```python
from build123d import *

# Parameters (mm, degrees)
SKETCH_1_W          = 250
SKETCH_1_H          = 250
SKETCH_1_W_2        = 206
SKETCH_1_H_2        = 84
EXTRUDE_1_DEPTH     = 5.8
CUT_EXTRUDE_1_REACH = 355.601
SKETCH_2_W          = 47.2
SKETCH_2_H          = 5.8
SKETCH_2_W_2        = 5.8
SKETCH_2_H_2        = 53


with BuildPart() as part:
    # Эскиз1 → Бобышка-Вытянуть1 (new body)
    with BuildSketch(Plane(origin=(0, 0, 0), x_dir=(1, 0, 0), z_dir=(0, 1, 0))):
        with Locations((125, 125)):
            Rectangle(SKETCH_1_W, SKETCH_1_H)
        with Locations((125, 186)):
            Rectangle(SKETCH_1_W_2, SKETCH_1_H_2, mode=Mode.SUBTRACT)
        with Locations((125, 64)):
            Rectangle(SKETCH_1_W_2, SKETCH_1_H_2, mode=Mode.SUBTRACT)
    extrude(amount=EXTRUDE_1_DEPTH)

    # Эскиз2 → Вырез-Вытянуть1 (cut, up to next)
    with BuildSketch(Plane(origin=(0, 5.8, 0), x_dir=(1, 0, 0), z_dir=(0, 1, 0)), mode=Mode.PRIVATE) as cut_extrude_1_sk1:
        with Locations((77.4, 2.9)):
            Rectangle(SKETCH_2_W, SKETCH_2_H)
    cut_extrude_1_tool1 = extrude(cut_extrude_1_sk1.sketch, amount=-CUT_EXTRUDE_1_REACH, mode=Mode.PRIVATE) & part.part
    # Эскиз2 → Вырез-Вытянуть1 (cut, up to next)
    with BuildSketch(Plane(origin=(0, 5.8, 0), x_dir=(1, 0, 0), z_dir=(0, 1, 0)), mode=Mode.PRIVATE) as cut_extrude_1_sk2:
        with Locations((77.4, 125)):
            Rectangle(SKETCH_2_W, SKETCH_2_H)
    cut_extrude_1_tool2 = extrude(cut_extrude_1_sk2.sketch, amount=-CUT_EXTRUDE_1_REACH, mode=Mode.PRIVATE) & part.part
    # Эскиз2 → Вырез-Вытянуть1 (cut, up to next)
    with BuildSketch(Plane(origin=(0, 5.8, 0), x_dir=(1, 0, 0), z_dir=(0, 1, 0)), mode=Mode.PRIVATE) as cut_extrude_1_sk3:
        with Locations((77.4, 247.1)):
            Rectangle(SKETCH_2_W, SKETCH_2_H)
    cut_extrude_1_tool3 = extrude(cut_extrude_1_sk3.sketch, amount=-CUT_EXTRUDE_1_REACH, mode=Mode.PRIVATE) & part.part
    # Эскиз2 → Вырез-Вытянуть1 (cut, up to next)
    with BuildSketch(Plane(origin=(0, 5.8, 0), x_dir=(1, 0, 0), z_dir=(0, 1, 0)), mode=Mode.PRIVATE) as cut_extrude_1_sk4:
        with Locations((2.9, 175.5)):
            Rectangle(SKETCH_2_W_2, SKETCH_2_H_2)
    cut_extrude_1_tool4 = extrude(cut_extrude_1_sk4.sketch, amount=-CUT_EXTRUDE_1_REACH, mode=Mode.PRIVATE) & part.part
    # Эскиз2 → Вырез-Вытянуть1 (cut, up to next)
    with BuildSketch(Plane(origin=(0, 5.8, 0), x_dir=(1, 0, 0), z_dir=(0, 1, 0)), mode=Mode.PRIVATE) as cut_extrude_1_sk5:
        with Locations((2.9, 74.5)):
            Rectangle(SKETCH_2_W_2, SKETCH_2_H_2)
    cut_extrude_1_tool5 = extrude(cut_extrude_1_sk5.sketch, amount=-CUT_EXTRUDE_1_REACH, mode=Mode.PRIVATE) & part.part
    # Эскиз2 → Вырез-Вытянуть1 (cut, up to next)
    with BuildSketch(Plane(origin=(0, 5.8, 0), x_dir=(1, 0, 0), z_dir=(0, 1, 0)), mode=Mode.PRIVATE) as cut_extrude_1_sk6:
        with Locations((172.6, 2.9)):
            Rectangle(SKETCH_2_W, SKETCH_2_H)
    cut_extrude_1_tool6 = extrude(cut_extrude_1_sk6.sketch, amount=-CUT_EXTRUDE_1_REACH, mode=Mode.PRIVATE) & part.part
    # Эскиз2 → Вырез-Вытянуть1 (cut, up to next)
    with BuildSketch(Plane(origin=(0, 5.8, 0), x_dir=(1, 0, 0), z_dir=(0, 1, 0)), mode=Mode.PRIVATE) as cut_extrude_1_sk7:
        with Locations((172.6, 125)):
            Rectangle(SKETCH_2_W, SKETCH_2_H)
    cut_extrude_1_tool7 = extrude(cut_extrude_1_sk7.sketch, amount=-CUT_EXTRUDE_1_REACH, mode=Mode.PRIVATE) & part.part
    # Эскиз2 → Вырез-Вытянуть1 (cut, up to next)
    with BuildSketch(Plane(origin=(0, 5.8, 0), x_dir=(1, 0, 0), z_dir=(0, 1, 0)), mode=Mode.PRIVATE) as cut_extrude_1_sk8:
        with Locations((172.6, 247.1)):
            Rectangle(SKETCH_2_W, SKETCH_2_H)
    cut_extrude_1_tool8 = extrude(cut_extrude_1_sk8.sketch, amount=-CUT_EXTRUDE_1_REACH, mode=Mode.PRIVATE) & part.part
    # Эскиз2 → Вырез-Вытянуть1 (cut, up to next)
    with BuildSketch(Plane(origin=(0, 5.8, 0), x_dir=(1, 0, 0), z_dir=(0, 1, 0)), mode=Mode.PRIVATE) as cut_extrude_1_sk9:
        with Locations((247.1, 175.5)):
            Rectangle(SKETCH_2_W_2, SKETCH_2_H_2)
    cut_extrude_1_tool9 = extrude(cut_extrude_1_sk9.sketch, amount=-CUT_EXTRUDE_1_REACH, mode=Mode.PRIVATE) & part.part
    # Эскиз2 → Вырез-Вытянуть1 (cut, up to next)
    with BuildSketch(Plane(origin=(0, 5.8, 0), x_dir=(1, 0, 0), z_dir=(0, 1, 0)), mode=Mode.PRIVATE) as cut_extrude_1_sk10:
        with Locations((247.1, 74.5)):
            Rectangle(SKETCH_2_W_2, SKETCH_2_H_2)
    cut_extrude_1_tool10 = extrude(cut_extrude_1_sk10.sketch, amount=-CUT_EXTRUDE_1_REACH, mode=Mode.PRIVATE) & part.part
    add(cut_extrude_1_tool1.solids().sort_by_distance((77.4, 5.8, -2.9))[0], mode=Mode.SUBTRACT)
    add(cut_extrude_1_tool2.solids().sort_by_distance((77.4, 5.8, -125))[0], mode=Mode.SUBTRACT)
    add(cut_extrude_1_tool3.solids().sort_by_distance((77.4, 5.8, -247.1))[0], mode=Mode.SUBTRACT)
    add(cut_extrude_1_tool4.solids().sort_by_distance((2.9, 5.8, -175.5))[0], mode=Mode.SUBTRACT)
    add(cut_extrude_1_tool5.solids().sort_by_distance((2.9, 5.8, -74.5))[0], mode=Mode.SUBTRACT)
    add(cut_extrude_1_tool6.solids().sort_by_distance((172.6, 5.8, -2.9))[0], mode=Mode.SUBTRACT)
    add(cut_extrude_1_tool7.solids().sort_by_distance((172.6, 5.8, -125))[0], mode=Mode.SUBTRACT)
    add(cut_extrude_1_tool8.solids().sort_by_distance((172.6, 5.8, -247.1))[0], mode=Mode.SUBTRACT)
    add(cut_extrude_1_tool9.solids().sort_by_distance((247.1, 5.8, -175.5))[0], mode=Mode.SUBTRACT)
    add(cut_extrude_1_tool10.solids().sort_by_distance((247.1, 5.8, -74.5))[0], mode=Mode.SUBTRACT)


solid = part.part
```
Could you check a few things on this model? Use its own coordinates, in mm. A direction names the side the tool comes from. Coordinates: 2 decimals unless noted, no trailing zeros. Loops run counter-clockwise (first coordinate to the right, second up) from the corner with the lowest first, then second, coordinate; pieces in that order, holes last. Notation, with made-up numbers: M 4,47 L 33,47 A28 cw 33,65 Z; hole C -27,-29 d8. An arc over 180 degrees is marked long. Put each result on its own line as item: value. Start each with the question number.
(1) For faces 4 (the face through (223, 3, 0)), 5 (the face through (172, 3, -5.8)), 6 (the face through (101, 3, -247)), 7 (the face through (77, 3, -122.1)), 8 (the face through (123, 5.8, -127)), which set-ups out of +Z, -Z, +X, -X, +Y, -Y let a thin tool reach every point of the face, with its end or its side?
(2) Suppose I cut it at C-C on x = 204.5. Please give me the cut outline in (y, z).
(3) Suppose I cut it at B-B on x = 165.5. Please give me the cut outline in (y, z).
(4) I need wall thicknesses on line 1 (Z direction, x = 61, y = 4.95); line 2 (Z direction, x = 125, y = 4.05); line 3 (X direction, y = 1.8, z = -61.5). Which ranges of each line are inside material? Lowest first, please. Write a range as from..to.
(5) Thinking about a two-plate mould opening in X: for faces 1 (the face through (250, 3, -24)), 2 (the face through (53.8, 3, -3)), 3 (the face through (125, 3, 0)), which applies, pulls with the +X half, pulls with the -X half, needs draft (parallel to the pull), parting line crosses it, or undercut?
(6) Will these pins go through, and if not, where does the flat tip stop? P1, Ø3, axis at y = 3.5, z = -176, coming from the -X side; P2, Ø1.7, axis at x = 180.5, y = 3.5, coming from the +Z side.
(7) Suppose I cut it at A-A on z = -34. Please give me the cut outline in (x, y).
(8) Suppose I cut it at D-D on z = -95.5. Please give me the cut outline in (x, y).
Solutions:
1. face 4: +Z, +X, -X, +Y, -Y
1. face 5: +Z, +Y, -Y
1. face 6: -Z, +Y, -Y
1. face 7: +Y, -Y
1. face 8: +Z, -Z, +X, -X, +Y
2. outline: M 0,-250 L 5.8,-250 L 5.8,-228 L 0,-228 Z; M 0,-144 L 5.8,-144 L 5.8,-106 L 0,-106 Z; M 0,-22 L 5.8,-22 L 5.8,0 L 0,0 Z
3. outline: M 0,-244.2 L 5.8,-244.2 L 5.8,-228 L 0,-228 Z; M 0,-144 L 5.8,-144 L 5.8,-127.9 L 0,-127.9 Z; M 0,-122.1 L 5.8,-122.1 L 5.8,-106 L 0,-106 Z; M 0,-22 L 5.8,-22 L 5.8,-5.8 L 0,-5.8 Z
4. line 1: z = -244.2..-228, -144..-127.9, -122.1..-106, -22..-5.8
4. line 2: z = -250..-228, -144..-106, -22..0
4. line 3: x = 5.8..22, 228..244.2
5. face 1: pulls with the +X half
5. face 2: undercut
5. face 3: needs draft
6. P1: stops at x = 5.8
6. P2: stops at z = -5.8
7. outline: M 0,0 L 22,0 L 22,5.8 L 0,5.8 Z; M 228,0 L 250,0 L 250,5.8 L 228,5.8 Z
8. outline: M 5.8,0 L 22,0 L 22,5.8 L 5.8,5.8 Z; M 228,0 L 244.2,0 L 244.2,5.8 L 228,5.8 Z
